Model file for the job. Use its own axes, mm. Round coordinates to 2 decimals unless told otherwise and drop trailing zeros. Order: outer loops, then holes, each group sorted by start corner. A loop starts at its lowest first (then second) coordinate and runs counter-clockwise, first axis right, second up. Notation, with made-up numbers: (-17, 48.25) -> (-9, 48.25) arc R32 cw to (-9, 77.25) -> close; hole circle Ø6 at (73.5, 34). An arc over 180 degrees is marked (long way). Use CSV: the item, a comma, the result in double quotes.
```python
from build123d import *

# Parameters (mm, degrees)
SKETCH1_W           = 114.3
SKETCH1_H           = 25.4
BOSS_EXTRUDE1_DEPTH = 6.35
CUT_EXTRUDE1_REACH  = 155.979
SKETCH2_R           = 12.7
SKETCH2_R_2         = 6.35


with BuildPart() as part:
    # Sketch1 → Boss-Extrude1 (new body)
    with BuildSketch(Plane(origin=(0, 0, 0), x_dir=(1, 0, 0), z_dir=(0, 1, 0))):
        with Locations((-57.15, 12.7)):
            Rectangle(SKETCH1_W, SKETCH1_H)
        Polygon((-88.9, 76.726438931), (0, 25.4), (-114.3, 25.4), (-114.3, 0), (-133.35, 32.995567884), align=None)
    extrude(amount=BOSS_EXTRUDE1_DEPTH)

    # Sketch2 → Cut-Extrude1 (cut, up to next)
    with BuildSketch(Plane.XZ, mode=Mode.PRIVATE) as cut_extrude1_sk1:
        with Locations(Location((-88.9, -25.4, 0), (0, 0, 270))):
            Circle(SKETCH2_R)
    cut_extrude1_tool1 = extrude(cut_extrude1_sk1.sketch, amount=-CUT_EXTRUDE1_REACH, mode=Mode.PRIVATE) & part.part
    # Sketch2 → Cut-Extrude1 (cut, up to next)
    with BuildSketch(Plane.XZ, mode=Mode.PRIVATE) as cut_extrude1_sk2:
        with Locations(Location((-25.4, -12.7, 0), (0, 0, 270))):
            Circle(SKETCH2_R_2)
    cut_extrude1_tool2 = extrude(cut_extrude1_sk2.sketch, amount=-CUT_EXTRUDE1_REACH, mode=Mode.PRIVATE) & part.part
    add(cut_extrude1_tool1.solids().sort_by_distance((-88.9, 0, -25.4))[0], mode=Mode.SUBTRACT)
    add(cut_extrude1_tool2.solids().sort_by_distance((-25.4, 0, -12.7))[0], mode=Mode.SUBTRACT)


solid = part.part
```
Q1. Cut at A-A (y = 3.5). Give the cut face in (x, z).
From the geometry:
outline,"(-133.35, -33) -> (-88.9, -76.73) -> (0, -25.4) -> (0, 0) -> (-114.3, 0) -> close; hole circle Ø25.4 at (-88.9, -25.4); hole circle Ø12.7 at (-25.4, -12.7)"
Q2. Cut at C-C (x = -81). Give the cut face in (y, z), plus the area to 3 significant figures.
From the geometry:
outline,"(0, -72.17) -> (6.35, -72.17) -> (6.35, -35.34) -> (0, -35.34) -> close; (0, -15.46) -> (6.35, -15.46) -> (6.35, 0) -> (0, 0) -> close"
area,"332 mm²"
Q3. Mould opens along X. For faces 1 (the cylindrical face through (-29.26, 3.13, -7.66)), 2 (the flat face through (-123.692, 3.131, -16.267)), 3 (the flat face through (0, 3, -13)), 4 (the cylindrical face through (-76.308, 3.131, -23.747)) say: +X half, -X half, draft (parallel to the pull), parting line (faces both ways), or undercut.
From the geometry:
face 1,"undercut"
face 2,"-X half"
face 3,"+X half"
face 4,"undercut"
Q4. Cut at D-D (z = -42.5). Give the cut face in (x, y).
From the geometry:
outline,"(-123.69, 0) -> (-29.62, 0) -> (-29.62, 6.35) -> (-123.69, 6.35) -> close"
Q5. Cut at B-B (z = -9.5). Give the cut face in (x, y), plus the area to 3 significant figures.
From the geometry:
outline,"(-119.78, 0) -> (-30.88, 0) -> (-30.88, 6.35) -> (-119.78, 6.35) -> close; (-19.92, 0) -> (0, 0) -> (0, 6.35) -> (-19.92, 6.35) -> close"
area,"691 mm²"
Q6. Probe line 1 along X through (y, z) = (1.75, -25.4); line 2 along Z through (x, y) = (-11, 4.5); line 3 along X through (y, z) = (3.5, -12). List the from-to ranges inside material, lowest first.
From the geometry:
line 1,"x = -128.96 to -101.6, -76.2 to 0"
line 2,"z = -31.75 to 0"
line 3,"x = -121.23 to -31.71, -19.09 to 0"
Q7. Pin check, flat tips, straight feed: pin 1 (3 mm diameter, centred on x = -18.5, y = 2, fed in from -Z); pin 2 (2 mm diameter, centred on y = 1, z = -24, fed in from -X). Stop position of each tip, or through.
From the geometry:
pin 1,"stops at z = -36.95"
pin 2,"stops at x = -128.73"
